CAD build for the part. Positions are in the model's coordinates, mm. A direction names the side the tool comes from. Round coordinates to 2 decimals unless told otherwise and drop trailing zeros. Loops run counter-clockwise (first coordinate to the right, second up) from the corner with the lowest first, then second, coordinate; pieces in that order, holes last. Notation, with made-up numbers: M -9.5,-3.75 L 5.5,-3.75 A22 ccw 5.5,18.25 Z; hole C 67,87 d7. An arc over 180 degrees is marked long. Use one line per item in the form item = value.
from build123d import *

# Parameters (mm, degrees)
F1_DEPTH = 7
F2_SIZE  = 2


with BuildPart() as f1:
    # F0 (on Top) → F1 (new body)
    with BuildSketch(Plane.XY):
        Polygon((-1, -7.4), (-1, 0), (-2.9, 0), (-2.9, -3.2000038773), (-2.9, -7.4), align=None)
        with BuildLine():
            Line((-2.9, 0), (-1, 0))
            Line((-1, 0), (1, 0))
            Line((1, 0), (2.9, 0))
            Line((2.9, 0), (4.15, 0))
            Line((4.15, 0), (4.15, -2))
            Line((4.15, -2), (5.65, -2))
            Line((5.65, -2), (5.65, 2.25))
            Line((5.65, 2.25), (-4.9, 12.8))
            Line((-4.9, 12.8), (-4.9, 35))
            Line((-4.9, 35), (-4.9, 38))
            Line((-4.9, 38), (-4.9, 50))
            Line((-4.9, 50), (7.1, 50))
            Line((7.1, 50), (10.1, 50))
            Line((10.1, 50), (14.5457633434, 50))
            Line((14.5457633434, 50), (21.060983901, 46.9619027594))
            ThreePointArc((21.060983901, 46.9619027594), (21.1916137331, 48.280211467), (22.1175295553, 49.227672227))
            Line((22.1175295553, 49.227672227), (15.1, 52.5))
            Line((15.1, 52.5), (-7.4, 52.5))
            Line((-7.4, 52.5), (-7.4, -2))
            Line((-7.4, -2), (-4.15, -2))
            Line((-4.15, -2), (-4.15, 0))
            Line((-4.15, 0), (-2.9, 0))
        make_face()
        Polygon((-4.9, 9.8), (2.65, 2.25), (-4.9, 2.25), align=None, mode=Mode.SUBTRACT)
        Polygon((2.9, 0), (1, 0), (1, -7.4), (2.9, -7.4), (2.9, -3.2000038773), align=None)
        Polygon((-2.9, -7.4), (-2.9, -3.2000038773), (-3.6, -4.3000019386), (-3.6, -6.3000019386), align=None)
        Polygon((3.6, -4.3000019386), (2.9, -3.2000038773), (2.9, -7.4), (3.6, -6.3000019386), align=None)
        with BuildLine():
            ThreePointArc((25.0042293071, 47.4349749436), (24.0593597485, 49.1340040051), (22.1175295553, 49.227672227))
            Line((22.1175295553, 49.227672227), (23.5325021343, 48.5678596774))
            Line((23.5325021343, 48.5678596774), (22.47595648, 46.3020902098))
            Line((22.47595648, 46.3020902098), (21.060983901, 46.9619027594))
            ThreePointArc((21.060983901, 46.9619027594), (23.2424615338, 45.4492142817), (25.0042293071, 47.4349749436))
        make_face()
        with BuildLine():
            Line((23.5325021343, 48.5678596774), (22.1175295553, 49.227672227))
            ThreePointArc((22.1175295553, 49.227672227), (21.1916137331, 48.280211467), (21.060983901, 46.9619027594))
            Line((21.060983901, 46.9619027594), (22.47595648, 46.3020902098))
            Line((22.47595648, 46.3020902098), (23.5325021343, 48.5678596774))
        make_face()
        Polygon((-4.9, 38), (-4.9, 35), (10.1, 50), (7.1, 50), align=None)
    extrude(amount=F1_DEPTH)

    # F2
    f2_edges = [f1.edges().sort_by_distance(p)[0] for p in [
        (-4.9, 50, 3.5),
        (-7.4, 52.5, 3.5),
        (-7.4, -2, 3.5),
    ]]
    chamfer(f2_edges, length=F2_SIZE)


solid = f1.part
1. Cut at B-B on z = 5.25. State how many separate pieces and enclosed holes the cut face has, and give its area (3 significant figures).
Completed:
separate_pieces = 1
enclosed_holes = 2
area = 342 mm2
2. Cut at A-A on y = 5.5. Write the cut outline in (x, z), and give its area (3 significant figures).
Completed:
outline = M -7.4,0 L -4.9,0 L -4.9,7 L -7.4,7 Z; M -0.6,0 L 2.4,0 L 2.4,7 L -0.6,7 Z
area = 38.5 mm2
3. Cut at D-D on x = 17. Write the cut outline in (y, z), and give its area (3 significant figures).
Completed:
outline = M 48.86,0 L 51.61,0 L 51.61,7 L 48.86,7 Z
area = 19.3 mm2
4. Cut at C-C on y = 33.5. Write the cut outline in (x, z).
Completed:
outline = M -7.4,0 L -4.9,0 L -4.9,7 L -7.4,7 Z
5. Probe line 1 along Y through (x, z) = (2, 6.25); line 2 along Y through (x, z) = (5, 1.25); line 3 along Y through (x, z) = (0, 0.5). List the from-to ranges inside material, lowest first. Write a range as from..to.
Completed:
line_1 = -7.4..2.25, 2.9..5.9, 41.9..44.9, 50..52.5
line_2 = -2..2.9, 44.9..47.9, 50..52.5
line_3 = 0..2.25, 4.9..7.9, 39.9..42.9, 50..52.5
6. Pull direction Y, two halves, no side cores. Call faces 1 (the face through (-7.4, 26, 3)), 2 (the face through (5, 52.5, 3)), 3 (the face through (-1.2, 6.1, 3.5)): +Y half, -Y half, draft (parallel to the pull), parting line (faces both ways), or undercut.
Completed:
face_1 = draft
face_2 = +Y half
face_3 = undercut
7. Drop flat-ended pins along their axis: P1, Ø1.3, axis at y = -1, z = 3, coming from the +X side; P2, Ø1.6, axis at y = -2, z = 4, coming from the -X side; P3, Ø1.2, axis at x = 5, z = 4, coming from the -Y side. Give the stop position or say it passes through.
Completed:
P1 = 5.65
P2 = -6.2
P3 = -2
8. Tool access for faces 4 (the face through (1, -4, 3)), 5 (the face through (-3.6, -5, 3)), 6 (the face through (-4.9, 24, 3)), 7 (the face through (-1, 2.25, 3)): list every direction of +Z, -Z, +X, -X, +Y, -Y with a clear straight run to the whole face (end or side of a thin tool).
Completed:
face_4 = +Z, -Z, -Y
face_5 = +Z, -Z, -X, -Y
face_6 = +Z, -Z, +X
face_7 = +Z, -Z
